```python
from build123d import *

# Parameters (mm, degrees)
SKETCH_1_W          = 10
SKETCH_1_H          = 10
SKETCH_1_W_2        = 8
SKETCH_1_H_2        = 8
EXTRUDE_1_DEPTH     = 41.5
SKETCH_2_R          = 1.6
CUT_EXTRUDE_1_DEPTH = 10


with BuildPart() as part:
    # ｽｹｯﾁ1 → 押し出し-薄板1 (new body)
    with BuildSketch(Plane.XY):
        Rectangle(SKETCH_1_W, SKETCH_1_H)
        Rectangle(SKETCH_1_W_2, SKETCH_1_H_2, mode=Mode.SUBTRACT)
    extrude(amount=EXTRUDE_1_DEPTH)

    # ｽｹｯﾁ2 → ｶｯﾄ - 押し出し1 (cut)
    with BuildSketch(Plane(origin=(0, 5, 0), x_dir=(1, 0, 0), z_dir=(0, 1, 0))):
        with BuildLine():
            ThreePointArc((1.6, -6.5), (1.13137085, -5.36862915), (0, -4.9))
            Line((0, -4.9), (0, -8.1))
            ThreePointArc((0, -8.1), (1.13137085, -7.63137085), (1.6, -6.5))
        make_face()
        with BuildLine():
            Line((0, -8.1), (0, -4.9))
            ThreePointArc((0, -4.9), (-1.6, -6.5), (0, -8.1))
        make_face()
        with BuildLine():
            ThreePointArc((1.6, -26.5), (1.13137085, -25.36862915), (0, -24.9))
            Line((0, -24.9), (0, -28.1))
            ThreePointArc((0, -28.1), (1.13137085, -27.63137085), (1.6, -26.5))
        make_face()
        with BuildLine():
            Line((0, -28.1), (0, -24.9))
            ThreePointArc((0, -24.9), (-1.6, -26.5), (0, -28.1))
        make_face()
        with Locations(Location((0, -36.5, 0), (0, 0, 270))):
            Circle(SKETCH_2_R)
    extrude(amount=-CUT_EXTRUDE_1_DEPTH, mode=Mode.SUBTRACT)


solid = part.part
```
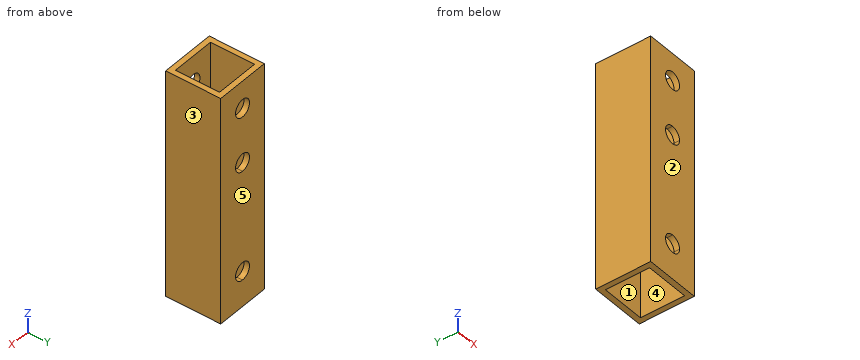
For this review, take the finished solid that the model builds, in its own axes (mm). Face numbers are marked on the shaded views. A direction names the side the tool comes from. Coordinates: 2 decimals unless noted, no trailing zeros. Write each loop counter-clockwise with the first axis right and the second up, starting at its lowest first coordinate (ties: lowest second). Pieces come first, ordered by that corner, then holes.
(1) Add section A-A on x = -2.5. Give the boundary of the cut face in (y, z).
(2) The part is to be moulded in two halves that separate along X. For the marked faces 3, 4 and 5, say which applies: +X half, -X half, draft (parallel to the pull), parting line (faces both ways), or undercut.
(3) Tool access review of the marked faces 1 and 2: name each direction out of +Z, -Z, +X, -X, +Y, -Y from which nothing blocks a thin tool from reaching the whole face with its end or side.
(4) Wall thickness on probe 1 along X at (y, z) = (3.25, 24); probe 2 along X at (y, z) = (-4.55, 36.5): over which ranges is each line inside the solid? List them lowest first.
(5) Add section C-C on z = 36.5. Give the boundary of the cut face in (x, y), then the cut area to 3 significant figures.
(6) Add section D-D on z = 22. Give the boundary of the cut face in (x, y), then the cut area to 3 significant figures.
Answer sheet:
1. outline: (-5, 0) - (-4, 0) - (-4, 41.5) - (-5, 41.5) - close; (4, 0) - (5, 0) - (5, 41.5) - (4, 41.5) - close
2. face 3: +X half
2. face 4: undercut
2. face 5: draft
3. face 1: +Z, -Z
3. face 2: +Z, -Z, +X, -X, -Y
4. probe 1: x = -5 to -4, 4 to 5
4. probe 2: x = -5 to -1.6, 1.6 to 5
5. outline: (-5, -5) - (-1.6, -5) - (-1.6, -4) - (-4, -4) - (-4, 4) - (-1.6, 4) - (-1.6, 5) - (-5, 5) - close; (1.6, -5) - (5, -5) - (5, 5) - (1.6, 5) - (1.6, 4) - (4, 4) - (4, -4) - (1.6, -4) - close
5. area: 29.6 mm2
6. outline: (-5, -5) - (5, -5) - (5, 5) - (-5, 5) - close; hole (-4, -4) - (4, -4) - (4, 4) - (-4, 4) - close
6. area: 36.0 mm2
